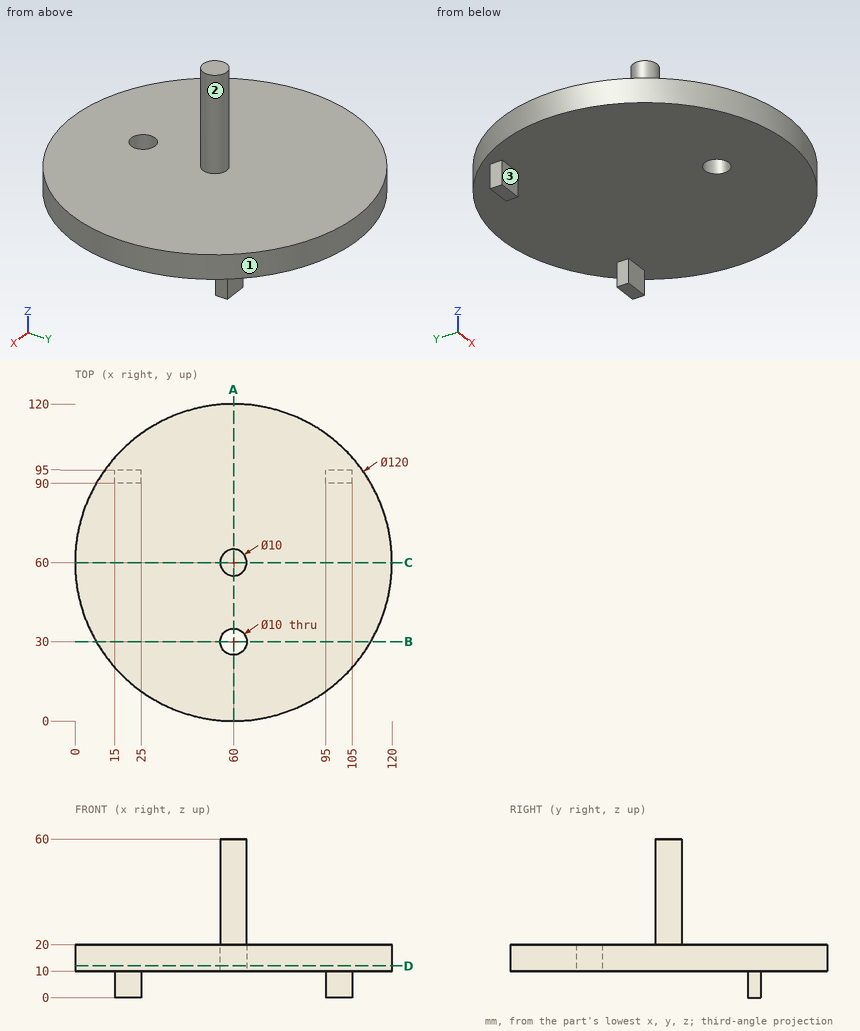
Job drawing, mm, ordinate dimensions from the low corner. One solid piece. A direction names the side the tool comes from. Give positions to 0.01 mm unless a question says otherwise; leave off trailing zeros. Write each loop counter-clockwise with the first axis right and the second up, starting at its lowest first coordinate (ties: lowest second). Pieces come first, ordered by that corner, then holes. Notation, with made-up numbers: (53.5, 50) - (69.5, 50) arc R6 cw to (69.5, 61) - close; hole circle Ø3 at (31, 53). An arc over 180 degrees is marked (long way). Use one line per item in the form item = value. Start each with the question number.
1. Band-saw the part on C-C on y = 60. Write the cut outline in (x, z).
2. Band-saw the part on A-A on x = 60. Write the cut outline in (y, z), plus the area to 3 significant figures.
3. Band-saw the part on D-D on z = 12. Write the cut outline in (x, y), plus the area to 3 significant figures.
4. 3-axis set-ups, long thin cutter, end or side, ignore diameter. For the marked faces 1, 2 and 3: which of +Z, -Z, +X, -X, +Y, -Y reach the whole face in a straight line?
5. Drop flat-ended pins along their axis: pin 1 Ø1 at (x, z) = (63, 35) entering from +Y; pin 2 Ø5 at (x, z) = (20, 7) entering from -Y; pin 3 Ø13 at (x, y) = (60, 30) entering from +Z. Give the stop position or say it passes through.
6. Band-saw the part on B-B on y = 30. Write the cut outline in (x, z), plus the area to 3 significant figures.
7. Probe line 1 (Y direction, x = 60, z = 12.5); line 2 (Z direction, x = 63, y = 47.5); line 3 (Y direction, x = 75, z = 18). List the from-to ranges inside material, lowest first. Write a range as [from, to].
Conclusion:
q1.outline = (0, 10) - (120, 10) - (120, 20) - (65, 20) - (65, 60) - (55, 60) - (55, 20) - (0, 20) - close
q2.outline = (0, 10) - (25, 10) - (25, 20) - (0, 20) - close; (35, 10) - (120, 10) - (120, 20) - (65, 20) - (65, 60) - (55, 60) - (55, 20) - (35, 20) - close
q2.area = 1,500 mm²
q3.outline = circle Ø120 at (60, 60); hole circle Ø10 at (60, 30)
q3.area = 11,200 mm²
q4.face_1 = +Z, -Z
q4.face_2 = +Z
q4.face_3 = -Z, +X, -X, -Y
q5.pin_1 = 64.33
q5.pin_2 = 90
q5.pin_3 = 20
q6.outline = (8.04, 10) - (55, 10) - (55, 20) - (8.04, 20) - close; (65, 10) - (111.96, 10) - (111.96, 20) - (65, 20) - close
q6.area = 939 mm²
q7.line_1 = [0, 25], [35, 120]
q7.line_2 = [10, 20]
q7.line_3 = [1.91, 118.09]
